CAD build for the part. Positions are in the model's coordinates, mm. A direction names the side the tool comes from. Coordinates: 2 decimals unless noted, no trailing zeros. Order: outer loops, then holes, each group sorted by start corner. A loop starts at its lowest first (then second) coordinate and runs counter-clockwise, first axis right, second up. Notation, with made-up numbers: M -11,27 L 14,27 A28 cw 14,53 Z; hole C -28.75,-13 d5. An arc over 180 degrees is marked long. One line per item, written item: value.
from build123d import *

# Parameters (mm, degrees)
SKETCH2_R           = 29.5
BOSS_EXTRUDE1_DEPTH = 7
SKETCH3_R           = 14
BOSS_EXTRUDE2_DEPTH = 3
SKETCH5_R           = 12.6
BOSS_EXTRUDE3_DEPTH = 8
SKETCH6_R           = 11
BOSS_EXTRUDE4_DEPTH = 34
SKETCH7_R           = 2.1
CUT_EXTRUDE1_DEPTH  = 33.8
SKETCH8_R           = 1.25
CUT_EXTRUDE2_DEPTH  = 19.2
SKETCH9_R           = 4.15
CUT_EXTRUDE3_DEPTH  = 9
SKETCH10_R          = 3.25
CUT_EXTRUDE4_DEPTH  = 3.5
SKETCH11_R          = 2.07
CUT_EXTRUDE5_DEPTH  = 4.5


with BuildPart() as part:
    # Sketch2 → Boss-Extrude1 (new body)
    with BuildSketch(Plane.XY):
        Circle(SKETCH2_R)
    extrude(amount=BOSS_EXTRUDE1_DEPTH)

    # Sketch3 → Boss-Extrude2 (add)
    with BuildSketch(Plane.XY.offset(7)):
        Circle(SKETCH3_R)
    extrude(amount=BOSS_EXTRUDE2_DEPTH)

    # Sketch5 → Boss-Extrude3 (add)
    with BuildSketch(Plane.XY.offset(10)):
        Circle(SKETCH5_R)
    extrude(amount=BOSS_EXTRUDE3_DEPTH)

    # Sketch6 → Boss-Extrude4 (add)
    with BuildSketch(Plane.XY.offset(18)):
        Circle(SKETCH6_R)
    extrude(amount=BOSS_EXTRUDE4_DEPTH)

    # Sketch7 → Cut-Extrude1 (cut)
    with BuildSketch(Plane(origin=(0, 0, 0), x_dir=(-1, 0, 0), z_dir=(0, 0, -1))):
        with Locations((8, 0)):
            Circle(SKETCH7_R)
        with Locations((5.656854249, -5.656854249)):
            Circle(SKETCH7_R)
        with Locations((0, -8)):
            Circle(SKETCH7_R)
        with Locations((-5.656854249, -5.656854249)):
            Circle(SKETCH7_R)
        with Locations((-8, 0)):
            Circle(SKETCH7_R)
        with Locations((-5.656854249, 5.656854249)):
            Circle(SKETCH7_R)
        with Locations((0, 8)):
            Circle(SKETCH7_R)
        with Locations((5.656854249, 5.656854249)):
            Circle(SKETCH7_R)
    extrude(amount=-CUT_EXTRUDE1_DEPTH, mode=Mode.SUBTRACT)

    # Sketch8 → Cut-Extrude2 (cut, through all)
    with BuildSketch(Plane(origin=(0, 0, 33.8), x_dir=(-1, 0, 0), z_dir=(0, 0, -1))):
        with Locations((-8, 0)):
            Circle(SKETCH8_R)
        with Locations((-5.656854249, 5.656854249)):
            Circle(SKETCH8_R)
        with Locations((0, 8)):
            Circle(SKETCH8_R)
        with Locations((5.656854249, 5.656854249)):
            Circle(SKETCH8_R)
        with Locations((8, 0)):
            Circle(SKETCH8_R)
        with Locations((5.656854249, -5.656854249)):
            Circle(SKETCH8_R)
        with Locations((0, -8)):
            Circle(SKETCH8_R)
        with Locations((-5.656854249, -5.656854249)):
            Circle(SKETCH8_R)
    extrude(amount=-CUT_EXTRUDE2_DEPTH, mode=Mode.SUBTRACT)

    # Sketch9 → Cut-Extrude3 (cut)
    with BuildSketch(Plane.XY.offset(52)):
        Circle(SKETCH9_R)
    extrude(amount=-CUT_EXTRUDE3_DEPTH, mode=Mode.SUBTRACT)

    # Sketch10 → Cut-Extrude4 (cut)
    with BuildSketch(Plane.XY.offset(7)):
        with Locations((-24.25, 0)):
            Circle(SKETCH10_R)
        with Locations((0, 24.25)):
            Circle(SKETCH10_R)
        with Locations((24.25, 0)):
            Circle(SKETCH10_R)
        with Locations((0, -24.25)):
            Circle(SKETCH10_R)
    extrude(amount=-CUT_EXTRUDE4_DEPTH, mode=Mode.SUBTRACT)

    # Sketch11 → Cut-Extrude5 (cut, through all)
    with BuildSketch(Plane.XY.offset(3.5)):
        with Locations((0, 24.25)):
            Circle(SKETCH11_R)
        with Locations((24.25, 0)):
            Circle(SKETCH11_R)
        with Locations((0, -24.25)):
            Circle(SKETCH11_R)
        with Locations((-24.25, 0)):
            Circle(SKETCH11_R)
    extrude(amount=-CUT_EXTRUDE5_DEPTH, mode=Mode.SUBTRACT)


solid = part.part
Q1. Slice it at A-A (x = -24.25). List the corners of the cut face in (y, z).
Recorded:
outline: M -16.8,0 L -2.07,0 L -2.07,3.5 L -3.25,3.5 L -3.25,7 L -16.8,7 Z; M 2.07,0 L 16.8,0 L 16.8,7 L 3.25,7 L 3.25,3.5 L 2.07,3.5 Z
Q2. Drill centre lines: line 1 along Y through (x, z) = (-0.5, 33); line 2 along X through (y, z) = (5, 21); line 3 along Z through (x, y) = (15, 15.5). Where is each one in solid material? Low to high.
Recorded:
line 1: y = -10.99 to -10.04, -5.96 to 5.96, 10.04 to 10.99
line 2: x = -9.8 to -7.65, -3.66 to 3.66, 7.65 to 9.8
line 3: z = 0 to 7
Q3. Slice it at C-C (z = 25). Give the number of separate pieces and of enclosed holes in the cut face, plus the area to 3 significant figures.
Recorded:
separate pieces: 1
enclosed holes: 8
area: 269 mm^2
Q4. Mould opens along X. For faces 4 (the face through (9.25, 0.05, 42.77)), 5 (the face through (0, 0, 0)), 6 (the face through (-0.9, -4.05, 47.56)) say: released by +X, released by -X, zero draft, split by the parting line, or undercut.
Recorded:
face 4: undercut
face 5: zero draft
face 6: undercut
Q5. Which spindle directions (+Z, -Z, +X, -X, +Y, -Y) get a long thin tool onto all of the face, cutting with end or side? Do faces 1 (the face through (5.08, 4.55, 42.77)), 2 (the face through (-13, 2, 10)), 3 (the face through (0.273, 10.082, 16.663)). Say none if no direction does.
Recorded:
face 1: +Z, -Z
face 2: +Z
face 3: -Z
Q6. Pin check, flat tips, straight feed: pin 1 Ø3 at (x, z) = (1.5, 13.5) entering from +Y; pin 2 Ø6 at (x, z) = (11, 6) entering from +Y; pin 3 Ø6 at (x, y) = (0, 24.25) entering from +Z. Stop position of each tip, or through.
Recorded:
pin 1: stops at y = 12.6
pin 2: stops at y = 28.39
pin 3: stops at z = 3.5
